Here's how the part is built. I have some questions about the finished solid (model axes, mm). Face numbers are marked on the shaded views. Give positions to 0.01 mm unless a question says otherwise; leave off trailing zeros. Order: outer loops, then holes, each group sorted by start corner. A loop starts at its lowest first (then second) coordinate and runs counter-clockwise, first axis right, second up. Notation, with made-up numbers: M 17,75 L 37,75 A22 ccw 37,86 Z; hole C 5,9 d8. An arc over 180 degrees is marked long. Use one line per item in the form item = value.
from build123d import *

# Parameters (mm, degrees)
F1_DEPTH = 40
F3_D     = 3.3
F5_D     = 4.2
F6_R     = 2
F9_DEPTH = 3


with BuildPart() as f1:
    # F0 (on Front) → F1 (new body)
    with BuildSketch(Plane.XZ):
        with BuildLine():
            Line((15, -6.1671362493), (25, -6.1671362493))
            Line((25, -6.1671362493), (25, 11.8328637507))
            Line((25, 11.8328637507), (-20, 11.8328637507))
            Line((-20, 11.8328637507), (-20, -6.1671362493))
            Line((-20, -6.1671362493), (-10, -6.1671362493))
            ThreePointArc((-10, -6.1671362493), (2.5, 6.3328637507), (15, -6.1671362493))
        make_face()
    extrude(amount=-F1_DEPTH)

    # F3 (through all)
    with Locations(Plane.XY.offset(11.8328637507)):
        with Locations((-12.5, 5), (-12.5, 35), (17.5, 35), (17.5, 5)):
            Hole(F3_D / 2)

    # F5 (through all)
    with Locations(Plane.XY.offset(11.8328637507)):
        with Locations((2.5, 20)):
            Hole(F5_D / 2)

    # F6
    f6_edges = [f1.edges().sort_by_distance(p)[0] for p in [
        (-20, 20, 11.832864),
        (25, 20, 11.832864),
    ]]
    fillet(f6_edges, radius=F6_R)


with BuildPart() as f9:
    # F8 (on Top) → F9 (new body)
    with BuildSketch(Plane.XY):
        Polygon((57.5, 170.0064360575), (30, 217.6378332657), (-30, 217.6378332657), (-57.5, 170.0064360575), (-57.5, 30.0064360575), (-40, -0.3044530749), (40, -0.3044530749), (57.5, 30.0064360575), align=None)
    extrude(amount=F9_DEPTH)


solid = f1.part
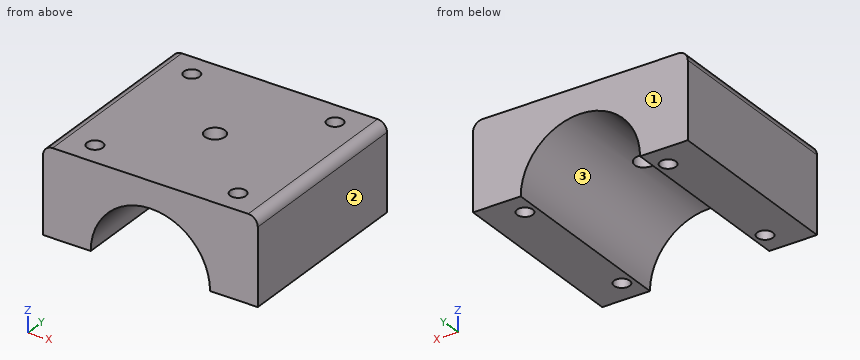
Q1. I want a section at B-B on z = 3.75. Write out the boundary of the cut face in (x, y).
Found:
outline = M -20,0 L -5.11,0 L -5.11,40 L -20,40 Z; M 10.11,0 L 25,0 L 25,40 L 10.11,40 Z; hole C -12.5,5 d3.3; hole C -12.5,35 d3.3; hole C 17.5,5 d3.3; hole C 17.5,35 d3.3
Q2. I want a section at A-A on y = 20. Write out the boundary of the cut face in (x, z).
Found:
outline = M -20,-6.17 L -10,-6.17 A12.5 cw 0.4,6.16 L 0.4,11.83 L -18,11.83 A2 ccw -20,9.83 Z; M 4.6,6.16 A12.5 cw 15,-6.17 L 25,-6.17 L 25,9.83 A2 ccw 23,11.83 L 4.6,11.83 Z
Q3. I want a section at C-C on x = 2.5. Write out the boundary of the cut face in (y, z).
Found:
outline = M 0,6.33 L 17.9,6.33 L 17.9,11.83 L 0,11.83 Z; M 22.1,6.33 L 40,6.33 L 40,11.83 L 22.1,11.83 Z
Q4. I want a section at D-D on y = 5. Write out the boundary of the cut face in (x, z), then the cut area to 3 significant figures.
Found:
outline = M -20,-6.17 L -14.15,-6.17 L -14.15,11.83 L -18,11.83 A2 ccw -20,9.83 Z; M -10.85,-6.17 L -10,-6.17 A12.5 cw 15,-6.17 L 15.85,-6.17 L 15.85,11.83 L -10.85,11.83 Z; M 19.15,-6.17 L 25,-6.17 L 25,9.83 A2 ccw 23,11.83 L 19.15,11.83 Z
area = 444 mm²
Q5. I need wall thicknesses on L1, parallel to Y at x = 17.5, z = 0; L2, parallel to X at y = 20, z = 8.7; L3, parallel to Y at x = -14, z = -3.5. Which ranges of each line are inside material? Lowest first, please.
Found:
L1 = 0 to 3.35, 6.65 to 33.35, 36.65 to 40
L2 = -20 to 0.4, 4.6 to 25
L3 = 0 to 4.31, 5.69 to 34.31, 35.69 to 40
Q6. Thinking about a two-plate mould opening in X: for the marked faces 1, 2 and 3, which applies, +X half, -X half, draft (parallel to the pull), parting line (faces both ways), or undercut?
Found:
face_1 = draft
face_2 = +X half
face_3 = undercut
